Input: part model. Units: mm. Frame: model coordinates. A direction names the side the tool comes from. Coordinates: 2 decimals unless noted, no trailing zeros. Loops run counter-clockwise (first coordinate to the right, second up) from the corner with the lowest first, then second, coordinate; pieces in that order, holes last. Notation, with made-up numbers: (73.25, 44) - (115.25, 44) arc R18 ccw to (115.25, 57) - close; hole circle Ø10 at (13.5, 66.5). An arc over 180 degrees is marked (long way). Use a Markdown table: item, result. Add a question column.
1. Section query A-A on y = 2. Return the cut outline in (x, z) (3 decimals), then the cut area to 3 significant figures.
2. Access query for faces 1 (the face through (17.75, 8, 7)), 2 (the face through (10, 12.5, 7)). Directions: +Z, -Z, +X, -X, +Y, -Y. A direction counts if a zero-diameter tool reaches every point of the face in a straight line with its end or side. Return the directions, or none.
3. Draft query along X for faces 3 (the face through (19.75, 6, 7)), 4 (the face through (10, 6, 15)), 5 (the face through (0, 6, 7)), 6 (the face through (8.277, 9.179, 3.93)). Return one class per face: released by +X, released by -X, zero draft, split by the parting line, or undercut.
4. Section query C-C on z = 11.5. Return the cut outline in (x, y) (3 decimals), then the cut area to 3 significant figures.
5. Section query D-D on y = 6.5. Return the cut outline in (x, z) (3 decimals), then the cut area to 3 significant figures.
6. Ray query, L1, parallel to X at y = 2.25, z = 4 (3 decimals); L2, parallel to Z at x = 8.5, y = 8.5; L3, parallel to Z at x = 10.5, y = 9.5. Return the intervals inside material, ascending. Write a range as [from, to].
7. Section query B-B on x = 5.5. Return the cut outline in (y, z), then the cut area to 3 significant figures.
```python
from build123d import *

# Parameters (mm, degrees)
SKETCH1_W           = 19.75
SKETCH1_H           = 12.5
BOSS_EXTRUDE1_DEPTH = 15
SKETCH2_R           = 1.6
CUT_EXTRUDE1_DEPTH  = 13.5
SKETCH3_W           = 19.75
SKETCH3_H           = 12.5
BOSS_EXTRUDE2_DEPTH = 2


with BuildPart() as part:
    # Sketch1 → Boss-Extrude1 (new body)
    with BuildSketch(Plane.XY):
        with Locations((9.875, 6.25)):
            Rectangle(SKETCH1_W, SKETCH1_H)
        with BuildLine():
            Line((17.75, 8.191371412), (17.75, 7))
            ThreePointArc((17.75, 7), (9.875, 4.766533398), (2, 7))
            Line((2, 7), (2, 8.191371412))
            ThreePointArc((2, 8.191371412), (9.875, 5.766533398), (17.75, 8.191371412))
        make_face(mode=Mode.SUBTRACT)
    extrude(amount=BOSS_EXTRUDE1_DEPTH)

    # Sketch2 → Cut-Extrude1 (cut, through all)
    with BuildSketch(Plane(origin=(0, 12.5, 0), x_dir=(1, 0, 0), z_dir=(0, 1, 0))):
        with Locations((9.875, -11.5)):
            Circle(SKETCH2_R)
        with Locations((9.875, -4)):
            Circle(SKETCH2_R)
    extrude(amount=-CUT_EXTRUDE1_DEPTH, mode=Mode.SUBTRACT)

    # Sketch3 → Boss-Extrude2 (add)
    with BuildSketch(Plane(origin=(0, 0, 0), x_dir=(-1, 0, 0), z_dir=(0, 0, -1))):
        with Locations((-9.875, 6.25)):
            Rectangle(SKETCH3_W, SKETCH3_H)
    extrude(amount=BOSS_EXTRUDE2_DEPTH)


solid = part.part
```
Resolved:
| question | item | result |
|---|---|---|
| 1 | outline | (0, -2) - (19.75, -2) - (19.75, 15) - (0, 15) - close; hole circle Ø3.2 at (9.875, 4); hole circle Ø3.2 at (9.875, 11.5) |
| 1 | area | 320 mm² |
| 2 | face 1 | +Z |
| 2 | face 2 | +Z, -Z, +X, -X, +Y |
| 3 | face 3 | released by +X |
| 3 | face 4 | zero draft |
| 3 | face 5 | released by -X |
| 3 | face 6 | undercut |
| 4 | outline | (0, 0) - (8.275, 0) - (8.275, 4.852) arc R15 cw to (2, 7) - (2, 8.191) arc R14 ccw to (8.275, 5.858) - (8.275, 12.5) - (0, 12.5) - close; (11.475, 0) - (19.75, 0) - (19.75, 12.5) - (11.475, 12.5) - (11.475, 5.858) arc R14 ccw to (17.75, 8.191) - (17.75, 7) arc R15 cw to (11.475, 4.852) - close |
| 4 | area | 193 mm² |
| 5 | outline | (0, -2) - (19.75, -2) - (19.75, 15) - (16.875, 15) - (16.875, 0) - (14.347, 0) - (14.347, 15) - (5.403, 15) - (5.403, 0) - (2.875, 0) - (2.875, 15) - (0, 15) - close; hole circle Ø3.2 at (9.875, 4); hole circle Ø3.2 at (9.875, 11.5) |
| 5 | area | 244 mm² |
| 6 | L1 | [0, 8.275], [11.475, 19.75] |
| 6 | L2 | [-2, 3.18], [4.82, 10.68], [12.32, 15] |
| 6 | L3 | [-2, 2.53], [5.47, 10.03], [12.97, 15] |
| 7 | outline | (0, -2) - (12.5, -2) - (12.5, 15) - (6.47, 15) - (6.47, 0) - (5.42, 0) - (5.42, 15) - (0, 15) - close |
| 7 | area | 197 mm² |
